from build123d import *

# Parameters (mm, degrees)
BOSS_EXTRU_1_DEPTH           = 3.5
ESQUISSE2_R                  = 2
ENL_V_MAT_EXTRU_1_DEPTH      = 395.382111663
ENL_V_MAT_EXTRU_2_DEPTH      = 395.382111663
ENL_V_MAT_EXTRU_2_DEPTH_BACK = 395.382111663
CONG_1_R                     = 5
ESQUISSE4_R                  = 1.5
ENL_V_MAT_EXTRU_3_DEPTH      = 309.078317965


with BuildPart() as part:
    # Esquisse1 → Boss.-Extru.1 (new body)
    with BuildSketch(Plane.XY):
        with BuildLine():
            Line((5, 0), (245, 0))
            ThreePointArc((245, 0), (248.535533906, 1.464466094), (250, 5))
            Line((250, 5), (250, 305))
            Line((250, 305), (0, 305))
            Line((0, 305), (0, 5))
            ThreePointArc((0, 5), (1.464466094, 1.464466094), (5, 0))
        make_face()
    extrude(amount=BOSS_EXTRU_1_DEPTH)

    # Esquisse2 → Enlèv. mat.-Extru.1 (cut, through all)
    with BuildSketch(Plane.XY.offset(3.5)):
        with Locations((5, 5)):
            Circle(ESQUISSE2_R)
        with Locations((245, 5)):
            Circle(ESQUISSE2_R)
        with Locations((5, 58.8)):
            Circle(ESQUISSE2_R)
        with Locations((245, 58.8)):
            Circle(ESQUISSE2_R)
    extrude(amount=-ENL_V_MAT_EXTRU_1_DEPTH, mode=Mode.SUBTRACT)

    # Esquisse3 → Enlèv. mat.-Extru.2 (cut, two sides: drawn at the far end of the back side and taken through both)
    with BuildSketch(Plane.XY.offset(3.5).offset(-ENL_V_MAT_EXTRU_2_DEPTH_BACK)):
        Polygon((-374.383398967, -414.136758554), (0, 110), (50, 180), (200, 180), (250, 110), (624.383398967, -414.136758554), (624.383398967, 874.090350445), (-374.383398967, 874.090350445), align=None)
    extrude(amount=ENL_V_MAT_EXTRU_2_DEPTH + ENL_V_MAT_EXTRU_2_DEPTH_BACK, mode=Mode.SUBTRACT)

    # Congé1
    cong_1_edges = [part.edges().sort_by_distance(p)[0] for p in [
        (50, 180, 1.75),
        (200, 180, 1.75),
        (250, 110, 1.75),
        (0, 110, 1.75),
    ]]
    fillet(cong_1_edges, radius=CONG_1_R)

    # Esquisse4 → Enlèv. mat.-Extru.3 (cut, through all)
    with BuildSketch(Plane(origin=(0, 0, 0), x_dir=(-1, 0, 0), z_dir=(0, 0, -1))):
        with Locations((-187, 20)):
            Circle(ESQUISSE4_R)
        with Locations((-187, 147)):
            Circle(ESQUISSE4_R)
        with Locations((-63, 147)):
            Circle(ESQUISSE4_R)
        with Locations((-63, 20)):
            Circle(ESQUISSE4_R)
    extrude(amount=-ENL_V_MAT_EXTRU_3_DEPTH, mode=Mode.SUBTRACT)


solid = part.part
Input: part model. Units: mm. Frame: model coordinates. Give positions to 0.01 mm unless a question says otherwise; leave off trailing zeros. Loops run counter-clockwise (first coordinate to the right, second up) from the corner with the lowest first, then second, coordinate; pieces in that order, holes last. Notation, with made-up numbers: (82.5, 74) - (137.5, 74) arc R23 cw to (137.5, 93) - close; hole circle Ø3 at (35, 13.25). An arc over 180 degrees is marked (long way). Use CSV: the item, a comma, the result in double quotes. Start each with the question number.
Item 1: Contact query for flat-ended pins moving along their axis: P1, Ø4.5, axis at x = 245, y = 58.8, coming from the +Z side; P2, Ø1.8, axis at x = 63, y = 147, coming from the -Z side; P3, Ø1, axis at y = 132, z = 2, coming from the -X side. Output: stop coordinate, or through.
Item 2: Section C-C on y = 134.5. Return loops of the section in (x, z), then the cut area to 4 significant figures.
Item 3: Section B-B on x = 224. Return loops of the section in (y, z).
Item 4: Section A-A on z = 1.15. State how many separate pieces and enclosed holes the cut face has, then the cut area to 3 significant figures.
Item 5: Line query: line 1 (Y direction, x = 187, z = 1.4); line 2 (X direction, y = 147, z = 2.1); line 3 (Y direction, x = 5, z = 0.95). Output: solid intervals per line, ascending.
Ans:
1,P1,"stops at z = 3.5"
1,P2,"passes through"
1,P3,"stops at x = 15.36"
2,outline,"(17.5, 0) - (232.5, 0) - (232.5, 3.5) - (17.5, 3.5) - close"
2,area,"752.5 mm2"
3,outline,"(0, 0) - (146.4, 0) - (146.4, 3.5) - (0, 3.5) - close"
4,separate pieces,"1"
4,enclosed holes,"8"
4,area,"41,400 mm2"
5,line 1,"y = 0 to 18.5, 21.5 to 145.5, 148.5 to 180"
5,line 2,"x = 26.43 to 61.5, 64.5 to 185.5, 188.5 to 223.57"
5,line 3,"y = 0 to 3, 7 to 56.8, 60.8 to 117"
